```python
from build123d import *

# Parameters (mm, degrees)
SKETCH2_W           = 35.4
SKETCH2_H           = 38.9
BOSS_EXTRUDE1_DEPTH = 1.5
SKETCH4_W           = 23.4
SKETCH4_H           = 12
CUT_EXTRUDE1_DEPTH  = 1.5
SKETCH5_W           = 35.4
SKETCH5_H           = 38.9
SKETCH5_W_2         = 29.4
SKETCH5_H_2         = 27.2
BOSS_EXTRUDE2_DEPTH = 10
FILLET1_R           = 5
SKETCH7_W           = 14.16
SKETCH7_H           = 5.2
CUT_EXTRUDE2_DEPTH  = 10
SKETCH8_W           = 7
SKETCH8_H           = 5.2
BOSS_EXTRUDE3_DEPTH = 1.8
BOSS_EXTRUDE4_DEPTH = 7.62
SKETCH10_R          = 0.95
BOSS_EXTRUDE5_DEPTH = 2
CHAMFER1_SIZE       = 1


with BuildPart() as part:
    # Sketch2 → Boss-Extrude1 (new body)
    with BuildSketch(Plane.XY):
        with Locations((0, 1.35)):
            Rectangle(SKETCH2_W, SKETCH2_H)
    extrude(amount=BOSS_EXTRUDE1_DEPTH)

    # Sketch4 → Cut-Extrude1 (cut)
    with BuildSketch(Plane(origin=(0, 0, 0), x_dir=(-1, 0, 0), z_dir=(0, 0, -1))):
        with Locations((0, 1.6)):
            Rectangle(SKETCH4_W, SKETCH4_H)
    extrude(amount=-CUT_EXTRUDE1_DEPTH, mode=Mode.SUBTRACT)

    # Sketch5 → Boss-Extrude2 (add)
    with BuildSketch(Plane(origin=(0, 0, 0), x_dir=(-1, 0, 0), z_dir=(0, 0, -1))):
        with Locations((0, 1.35)):
            Rectangle(SKETCH5_W, SKETCH5_H)
        Rectangle(SKETCH5_W_2, SKETCH5_H_2, mode=Mode.SUBTRACT)
    extrude(amount=BOSS_EXTRUDE2_DEPTH)

    # Fillet1
    fillet1_edges = [part.edges().sort_by_distance(p)[0] for p in [
        (-17.7, 20.8, -4.25),
        (17.7, 20.8, -4.25),
        (17.7, -18.1, -4.25),
        (-17.7, -18.1, -4.25),
    ]]
    fillet(fillet1_edges, radius=FILLET1_R)

    # Sketch7 → Cut-Extrude2 (cut)
    with BuildSketch(Plane(origin=(0, 0, -10), x_dir=(-1, 0, 0), z_dir=(0, 0, -1))):
        with Locations((0, 16.2)):
            Rectangle(SKETCH7_W, SKETCH7_H)
    extrude(amount=-CUT_EXTRUDE2_DEPTH, mode=Mode.SUBTRACT)

    # Sketch8 → Boss-Extrude3 (add)
    with BuildSketch(Plane(origin=(0, 0, 0), x_dir=(-1, 0, 0), z_dir=(0, 0, -1))):
        with Locations((11.2, -11)):
            Rectangle(SKETCH8_W, SKETCH8_H)
        with Locations((11.2, 11)):
            Rectangle(SKETCH8_W, SKETCH8_H)
        with Locations((-11.2, 11)):
            Rectangle(SKETCH8_W, SKETCH8_H)
        with Locations((-11.2, -11)):
            Rectangle(SKETCH8_W, SKETCH8_H)
    extrude(amount=BOSS_EXTRUDE3_DEPTH)

    # Sketch9 → Boss-Extrude4 (add)
    with BuildSketch(Plane(origin=(-14.7, 0, 0), x_dir=(0, 0, -1), z_dir=(1, 0, 0))):
        Polygon((3.5, 13.6), (10, 12.6), (10, 13.6), align=None)
    boss_extrude4 = extrude(amount=BOSS_EXTRUDE4_DEPTH)

    # Mirror1: Boss-Extrude4 across plane
    add(boss_extrude4.mirror(Plane(origin=(0, 0, 0), x_dir=(0, 0, 1), z_dir=(1, 0, 0))))

    # Sketch10 → Boss-Extrude5 (add)
    with BuildSketch(Plane(origin=(0, 0, -1.8), x_dir=(-1, 0, 0), z_dir=(0, 0, -1))):
        with Locations(Location((10.2, -12, 0), (0, 0, 180))):
            Circle(SKETCH10_R)
    boss_extrude5 = extrude(amount=BOSS_EXTRUDE5_DEPTH)

    # Mirror2: Boss-Extrude5 across plane
    add(boss_extrude5.mirror(Plane(origin=(0, 0, 0), x_dir=(0, 0, 1), z_dir=(1, 0, 0))))

    # Chamfer1
    chamfer1_edges = [part.edges().sort_by_distance(p)[0] for p in [
        (-11.7, 1.6, 1.5),
        (0, -4.4, 1.5),
        (11.7, 1.6, 1.5),
        (0, 7.6, 1.5),
    ]]
    chamfer(chamfer1_edges, length=CHAMFER1_SIZE)


solid = part.part
```
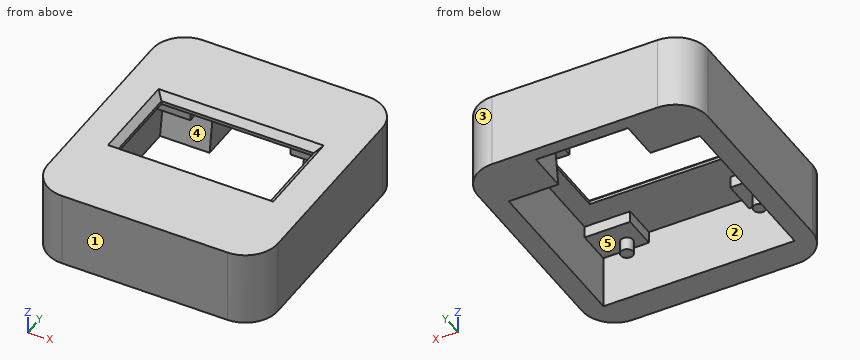
Build history of the part. All positions in model axes, mm. Face numbers are marked on the shaded views. A direction names the side the tool comes from. Coordinates: 2 decimals unless noted, no trailing zeros. Write each loop counter-clockwise with the first axis right and the second up, starting at its lowest first coordinate (ties: lowest second). Pieces come first, ordered by that corner, then holes.
1. Band-saw the part on C-C, the plane z = -1. Give the cut face in (x, y).
Answer block:
outline: (-17.7, -13.1) arc R5 ccw to (-12.7, -18.1) - (12.7, -18.1) arc R5 ccw to (17.7, -13.1) - (17.7, 15.8) arc R5 ccw to (12.7, 20.8) - (-12.7, 20.8) arc R5 ccw to (-17.7, 15.8) - close; hole (-14.7, -8.4) - (-7.7, -8.4) - (-7.7, -13.6) - (7.7, -13.6) - (7.7, -8.4) - (14.7, -8.4) - (14.7, 8.4) - (7.7, 8.4) - (7.7, 13.6) - (7.08, 13.6) - (7.08, 18.8) - (-7.08, 18.8) - (-7.08, 13.6) - (-7.7, 13.6) - (-7.7, 8.4) - (-14.7, 8.4) - close
2. Drop flat-ended pins along their axis: pin 1 (9 mm diameter, centred on x = 3.5, y = -5.5, fed in from -Z); pin 2 (1.5 mm diameter, centred on x = -10.5, y = -12, fed in from -Z); pin 3 (2.5 mm diameter, centred on x = 12, y = 12, fed in from -Z). Give the stop position or say it passes through.
Answer block:
pin 1: stops at z = 0
pin 2: stops at z = -3.8
pin 3: stops at z = -10
3. 3-axis set-ups, long thin cutter, end or side, ignore diameter. For the marked faces 1 and 2: which of +Z, -Z, +X, -X, +Y, -Y reach the whole face in a straight line?
Answer block:
face 1: +Z, -Z, +X, -X, -Y
face 2: -Z
4. Band-saw the part on B-B, the plane x = -10.2. Give the cut face in (y, z).
Answer block:
outline: (-18.1, -10) - (-13.6, -10) - (-13.6, -1.8) - (-12.95, -1.8) - (-12.95, -3.8) - (-11.05, -3.8) - (-11.05, -1.8) - (-8.4, -1.8) - (-8.4, 0) - (-4.4, 0) - (-4.4, 0.5) - (-5.4, 1.5) - (-18.1, 1.5) - close; (7.6, 0) - (8.4, 0) - (8.4, -1.8) - (13.6, -1.8) - (13.6, -3.5) - (12.6, -10) - (20.8, -10) - (20.8, 1.5) - (8.6, 1.5) - (7.6, 0.5) - close
5. Band-saw the part on D-D, the plane y = -10.5. Give the cut face in (x, z), and give its area (3 significant figures).
Answer block:
outline: (-17.7, -10) - (-14.7, -10) - (-14.7, -1.8) - (-7.7, -1.8) - (-7.7, 0) - (7.7, 0) - (7.7, -1.8) - (14.7, -1.8) - (14.7, -10) - (17.7, -10) - (17.7, 1.5) - (-17.7, 1.5) - close
area: 138 mm2
6. Band-saw the part on A-A, the plane y = -2.5. Give the cut face in (x, z).
Answer block:
outline: (-17.7, -10) - (-14.7, -10) - (-14.7, 0) - (-11.7, 0) - (-11.7, 0.5) - (-12.7, 1.5) - (-17.7, 1.5) - close; (11.7, 0) - (14.7, 0) - (14.7, -10) - (17.7, -10) - (17.7, 1.5) - (12.7, 1.5) - (11.7, 0.5) - close
7. Drill centre lines: probe 1 along Y at (x, z) = (-10.5, -0.25); probe 2 along X at (y, z) = (2.5, -6); probe 3 along X at (y, z) = (15.5, -2.5). Where is each one in solid material? Low to high.
Answer block:
probe 1: y = -18.1 to -8.4, 8.4 to 20.8
probe 2: x = -17.7 to -14.7, 14.7 to 17.7
probe 3: x = -17.7 to -7.08, 7.08 to 17.7
8. Pull direction Z, two halves, no side cores. Call the marked faces 3, 4 and 5: released by +Z, released by -Z, zero draft, split by the parting line, or undercut.
Answer block:
face 3: zero draft
face 4: undercut
face 5: released by -Z
